from build123d import *

# Parameters (mm, degrees)
SKETCH1_W           = 40
SKETCH1_H           = 13
BOSS_EXTRUDE1_DEPTH = 6
SKETCH2_W           = 6
SKETCH2_H           = 2
CUT_EXTRUDE1_DEPTH  = 25.596747752
SKETCH3_R           = 0.8
CUT_EXTRUDE2_DEPTH  = 2
SKETCH4_W           = 32
SKETCH4_H           = 7
CUT_EXTRUDE3_DEPTH  = 22.868927729
FILLET1_R           = 4
FILLET3_R           = 6
SKETCH5_R           = 1.5
CUT_EXTRUDE4_DEPTH  = 2


with BuildPart() as part:
    # Sketch1 → Boss-Extrude1 (new body)
    with BuildSketch(Plane(origin=(0, 0, 0), x_dir=(1, 0, 0), z_dir=(0, 1, 0))):
        Rectangle(SKETCH1_W, SKETCH1_H)
    extrude(amount=BOSS_EXTRUDE1_DEPTH)

    # Sketch2 → Cut-Extrude1 (cut, through all)
    with BuildSketch(Plane.XY.offset(6.5)):
        with Locations((-17, 3)):
            Rectangle(SKETCH2_W, SKETCH2_H)
    extrude(amount=-CUT_EXTRUDE1_DEPTH, mode=Mode.SUBTRACT)

    # Sketch3 → Cut-Extrude2 (cut)
    with BuildSketch(Plane(origin=(0, 6, 0), x_dir=(1, 0, 0), z_dir=(0, 1, 0))):
        with Locations(Location((-17, 4, 0), (0, 0, 270))):
            Circle(SKETCH3_R)
        with Locations(Location((-17, -4, 0), (0, 0, 270))):
            Circle(SKETCH3_R)
    extrude(amount=-CUT_EXTRUDE2_DEPTH, mode=Mode.SUBTRACT)

    # Sketch4 → Cut-Extrude3 (cut, through all)
    with BuildSketch(Plane(origin=(0, 6, 0), x_dir=(1, 0, 0), z_dir=(0, 1, 0))):
        with Locations((4, -3)):
            Rectangle(SKETCH4_W, SKETCH4_H)
    extrude(amount=-CUT_EXTRUDE3_DEPTH, mode=Mode.SUBTRACT)

    # Fillet1
    fillet1_edges = [part.edges().sort_by_distance(p)[0] for p in [
        (-12, 3, -0.5),
    ]]
    fillet(fillet1_edges, radius=FILLET1_R)

    # Fillet3
    fillet3_edges = [part.edges().sort_by_distance(p)[0] for p in [
        (20, 3, -6.5),
    ]]
    fillet(fillet3_edges, radius=FILLET3_R - 0.0001)  # a hair under: the kernel refuses the full size

    # Sketch5 → Cut-Extrude4 (cut)
    with BuildSketch(Plane(origin=(0, 2, 0), x_dir=(1, 0, 0), z_dir=(0, 1, 0))):
        with Locations(Location((-17, 4, 0), (0, 0, 270))):
            Circle(SKETCH5_R)
        with Locations(Location((-17, -4, 0), (0, 0, 270))):
            Circle(SKETCH5_R)
    extrude(amount=-CUT_EXTRUDE4_DEPTH, mode=Mode.SUBTRACT)


solid = part.part
Read the model definition and answer for the solid it produces. Units are mm, in the model's axes. A direction names the side the tool comes from. Give positions to 0.01 mm unless a question says otherwise; leave off trailing zeros. Write each loop counter-clockwise with the first axis right and the second up, starting at its lowest first coordinate (ties: lowest second). Pieces come first, ordered by that corner, then holes. Notation, with made-up numbers: (13, 23) - (67, 23) arc R20 cw to (67, 42) - close; hole circle Ø4 at (77.5, 25). An arc over 180 degrees is marked (long way). Use CSV: the item, a comma, the result in double quotes. Start each with the question number.
(1) Determine the mould class of faces 1 (the cylindrical face through (18.289, 3.042, -4.696)), 2 (the cylindrical face through (-10.797, 2.958, 0.641)), 3 (the flat face through (-12, 3, 5)), 4 (the cylindrical face through (-17.78, 5.01, 3.83)) for opening direction Z: +Z half, -Z half, draft (parallel to the pull), parting line (faces both ways), or undercut.
(2) Consider line 1 along Z through (x, y) = (-17.5, 4.95); line 2 along Y through (x, z) = (-18, 0.25); line 3 along X through (y, z) = (1.1, 4). Determine where each line is inside the solid, lowest interval first.
(3) Given P1, Ø2, axis at x = 9.5, z = 1, coming from the -Y side; P2, Ø1.8, axis at x = -17, z = -4, coming from the -Y side; P3, Ø2, axis at x = -10.5, y = 3.5, coming from the +Z side; P4, Ø3, axis at x = -2, y = 3, coming from the +Z side, each flat-ended and moving along its own axis, determine where each tip first touches the part or whether it passes through.
(4) Find section B-B (x = -17). Give the vertices of the cut face in (y, z).
(5) For faces 5 (the flat face through (-17, 4, 0)), 6 (the cylindrical face through (-16.55, 1.01, 5.43)), 7 (the flat face through (6, 3, -0.5)), determine the directions among +Z, -Z, +X, -X, +Y, -Y from which every point of the face is accessible in a straight line to the end or side of a thin tool.
(6) Find section A-A (z = 4). Give the vertices of the cut face in (x, y).
(7) Find section C-C (y = 0.8). Count the separate pieces of the cut face and the enclosed holes in it, plus the area to 3 significant figures.
Findings below:
1,face 1,"-Z half"
1,face 2,"+Z half"
1,face 3,"draft"
1,face 4,"undercut"
2,line 1,"-6.5 to -4.62, -3.38 to 3.38, 4.62 to 6.5"
2,line 2,"0 to 2, 4 to 6"
2,line 3,"-20 to -18.5, -15.5 to -12"
3,P1,"through"
3,P2,"y = 4"
3,P3,"z = 1.56"
3,P4,"z = -0.5"
4,outline,"(0, -6.5) - (2, -6.5) - (2, -5.5) - (0, -5.5) - close; (0, -2.5) - (2, -2.5) - (2, 2.5) - (0, 2.5) - close; (0, 5.5) - (2, 5.5) - (2, 6.5) - (0, 6.5) - close; (4, -6.5) - (6, -6.5) - (6, -4.8) - (4, -4.8) - close; (4, -3.2) - (6, -3.2) - (6, 3.2) - (4, 3.2) - close; (4, 4.8) - (6, 4.8) - (6, 6.5) - (4, 6.5) - close"
5,face 5,"+Z, -Z, -X"
5,face 6,"-Y"
5,face 7,"+Z, +X, +Y, -Y"
6,outline,"(-20, 0) - (-18.5, 0) - (-18.5, 2) - (-20, 2) - close; (-20, 4) - (-17.8, 4) - (-17.8, 6) - (-20, 6) - close; (-16.2, 4) - (-14, 4) - (-14, 2) - (-15.5, 2) - (-15.5, 0) - (-12, 0) - (-12, 6) - (-16.2, 6) - close"
7,separate pieces,"1"
7,enclosed holes,"2"
7,area,"278 mm2"
